Verification items for the finished model (mm, model axes). A direction names the side the tool comes from. Give positions to 0.01 mm unless a question says otherwise; leave off trailing zeros. Loops run counter-clockwise (first coordinate to the right, second up) from the corner with the lowest first, then second, coordinate; pieces in that order, holes last. Notation, with made-up numbers: (-36.75, 29.5) - (-9.75, 29.5) arc R6 ccw to (-9.75, 37.5) - close; hole circle Ø9 at (12.25, -35). An arc over 180 degrees is marked (long way). One line per item, written item: value. Start each with the question number.
1. Gauge pin test, flat ends, axial feed: pin 1 (5 mm diameter, centred on y = 11, z = 35.5, fed in from +X); pin 2 (6 mm diameter, centred on x = 122.5, y = 12.5, fed in from -Z); pin 3 (4 mm diameter, centred on x = 50, y = 17, fed in from +Z). Record the tip position at first contact, or that the pin passes through.
2. Access from +Z, -Z, +X, -X, +Y, -Y to the whole of each face (thin tool, end or side, straight path). Record for faces 1 (the flat face through (-102, 10, -30)), 2 (the flat face through (112, 10, -10)), 3 (the flat face through (-112, 10, -10)), 4 (the flat face through (103, 10, 30)), 5 (the flat face through (-103, 10, 30)).
3. Sectioned sample at C-C (x = -56). Record the cut outline in (y, z), plus the area to 3 significant figures.
4. Sectioned sample at A-A (z = 0). Record the cut outline in (x, y).
5. Scan lines: L1, parallel to X at y = 4, z = 0; L2, parallel to Z at x = 117.5, y = 14.5; L3, parallel to Z at x = -1, y = 17. Record each from-to range of solid material in increasing order. Write a range as [from, to].
6. Mould release check, pull along Z, two halves, no side actions. Record for faces 6 (the cylindrical face through (-144.297, 10.14, 23.986)), 7 (the flat face through (102, 10, -30)), 8 (the cylindrical face through (58.573, 10.14, -13.007)): pulls with the +Z half, pulls with the -Z half, needs draft (parallel to the pull), parting line crosses it, or undercut.
from build123d import *
from build123d.topology import SkipClean

# Parameters (mm, degrees)
BOSS_EXTRUDE1_DEPTH = 20
SKETCH2_W           = 75
SKETCH2_H           = 20
CUT_EXTRUDE1_DEPTH  = 20
FILLET1_R           = 10
FILLET2_R           = 20


with BuildPart() as part:
    # Sketch1 → Boss-Extrude1 (new body)
    with BuildSketch(Plane(origin=(0, 0, 0), x_dir=(1, 0, 0), z_dir=(0, 1, 0))):
        with BuildLine():
            Line((68.738635424, 30), (150, 30))
            Line((150, 30), (150, -30))
            Line((150, -30), (68.738635424, -30))
            ThreePointArc((68.738635424, -30), (41.079191813, -62.74950199), (0, -75))
            Line((0, -75), (0, 75))
            ThreePointArc((0, 75), (41.079191813, 62.74950199), (68.738635424, 30))
        make_face()
    boss_extrude1 = extrude(amount=BOSS_EXTRUDE1_DEPTH)

    # Sketch2 → Cut-Extrude1 (cut)
    with BuildSketch(Plane(origin=(0, 20, 0), x_dir=(1, 0, 0), z_dir=(0, 1, 0))):
        with BuildLine():
            Line((0, 60), (0, -60))
            ThreePointArc((0, -60), (60, 0), (0, 60))
        make_face()
        with Locations((112.5, 0)):
            Rectangle(SKETCH2_W, SKETCH2_H)
    cut_extrude1 = extrude(amount=-CUT_EXTRUDE1_DEPTH, mode=Mode.SUBTRACT)

    # Mirror1: Boss-Extrude1, Cut-Extrude1 across plane
    with SkipClean():  # the faces are left unmerged after this step: merging them gives an invalid solid
        add(boss_extrude1.mirror(Plane(origin=(0, 0, 0), x_dir=(0, 0, 1), z_dir=(1, 0, 0))))
        add(cut_extrude1.mirror(Plane(origin=(0, 0, 0), x_dir=(0, 0, 1), z_dir=(1, 0, 0))), mode=Mode.SUBTRACT)
    add(part.part.scale(1), mode=Mode.REPLACE)  # the faces are merged on a copy

    # Fillet1
    fillet1_edges = [part.edges().sort_by_distance(p)[0] for p in [
        (68.738635424, 10, -30),
        (68.738635424, 10, 30),
        (-68.738635424, 10, -30),
        (-68.738635424, 10, 30),
    ]]
    fillet(fillet1_edges, radius=FILLET1_R)

    # Fillet2
    fillet2_edges = [part.edges().sort_by_distance(p)[0] for p in [
        (-150, 10, 30),
        (-150, 10, -30),
        (150, 10, -30),
        (150, 10, 30),
    ]]
    fillet(fillet2_edges, radius=FILLET2_R - 0.0001)  # a hair under: the kernel refuses the full size


solid = part.part
Results are:
1. pin 1: stops at x = 67.86
1. pin 2: stops at z = -30
1. pin 3: stops at z = 57.63
2. face 1: -Z, -X, +Y, -Y
2. face 2: +X, +Y, -Y
2. face 3: -X, +Y, -Y
2. face 4: +Z, +X, +Y, -Y
2. face 5: +Z, -X, +Y, -Y
3. outline: (0, -49.89) - (20, -49.89) - (20, -21.54) - (0, -21.54) - close; (0, 21.54) - (20, 21.54) - (20, 49.89) - (0, 49.89) - close
3. area: 1,130 mm^2
4. outline: (-75, 0) - (-60, 0) - (-60, 20) - (-75, 20) - close; (60, 0) - (75, 0) - (75, 20) - (60, 20) - close
5. L1: x = [-75, -60], [60, 75]
5. L2: z = [-30, -10], [10, 30]
5. L3: z = [-74.99, -59.99], [59.99, 74.99]
6. face 6: pulls with the +Z half
6. face 7: pulls with the -Z half
6. face 8: undercut
